Verification items for this drawing (mm, ordinates from the low corner). A direction names the side the tool comes from. Coordinates: 2 decimals unless noted, no trailing zeros. Loops run counter-clockwise (first coordinate to the right, second up) from the corner with the lowest first, then second, coordinate; pieces in that order, holes last. Notation, with made-up numbers: M 25,-33.75 L 43,-33.75 A16 ccw 43,-10.75 Z; hole C 66,-27 d6. An arc over 180 degrees is marked long. Return JSON: item names as keys, results as strings.
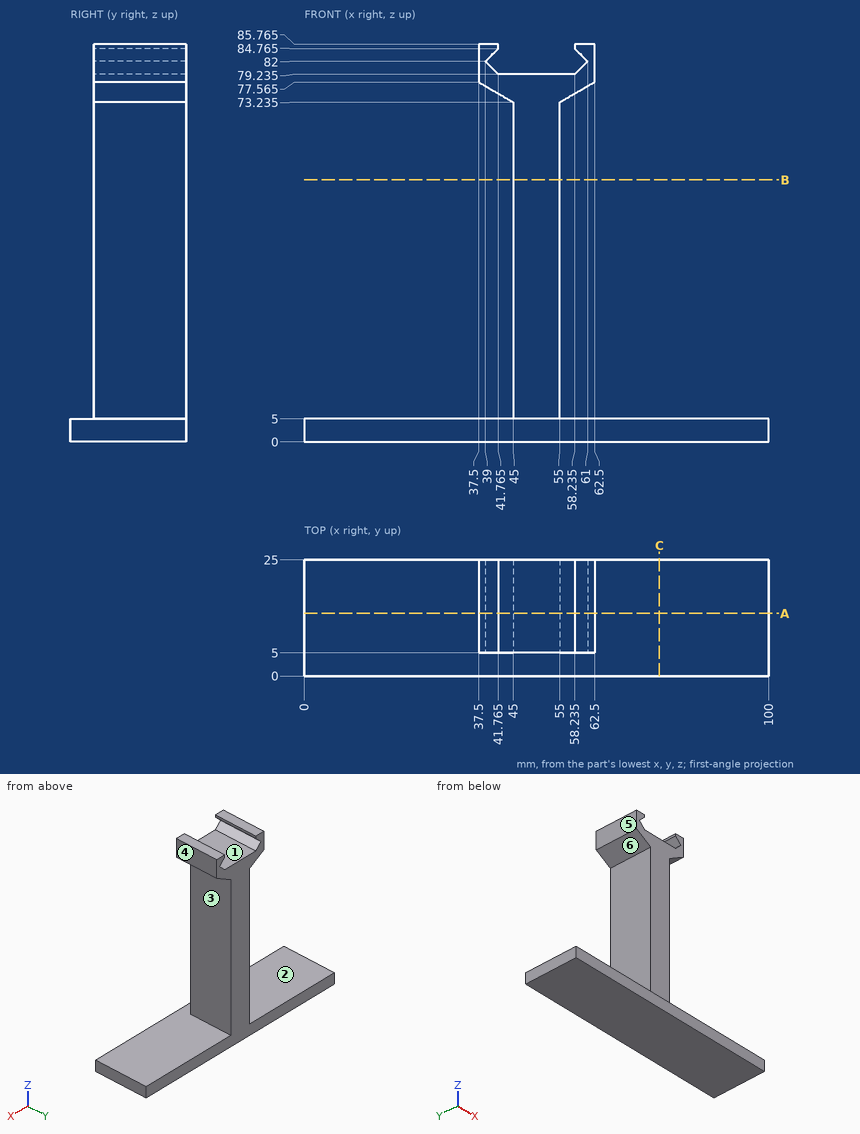
1) Section check A-A on y = 13.5. Record the cut outline in (x, z) (3 decimals).
Answers:
{"outline": "M 0,0 L 100,0 L 100,5 L 55,5 L 55,73.235 L 62.5,77.565 L 62.5,85.765 L 58.235,85.765 L 58.235,84.765 L 61,82 L 58.235,79.235 L 41.765,79.235 L 39,82 L 41.765,84.765 L 41.765,85.765 L 37.5,85.765 L 37.5,77.565 L 45,73.235 L 45,5 L 0,5 Z"}
2) Scan lines: line 1 along Y through (x, z) = (50, 62); line 2 along Z through (x, y) = (78, 22.25); line 3 along X through (y, z) = (9, 13.5). Record each from-to range of solid material in increasing order. Write a range as [from, to].
Answers:
{"line 1": "[5, 25]", "line 2": "[0, 5]", "line 3": "[45, 55]"}
3) Go/stop test with flat-tipped pins: pin 1 Ø6 at (y, z) = (21.5, 22.5) entering from +X; pin 2 Ø6 at (y, z) = (11, 76) entering from +X; pin 3 Ø0.5 at (y, z) = (11.5, 85.5) entering from -X. Record where each tip stops, or that it passes through.
Answers:
{"pin 1": "x = 55", "pin 2": "x = 62.5", "pin 3": "x = 37.5"}
4) Set-up check for the marked faces 4, 5 and 6: record each of +Z, -Z, +X, -X, +Y, -Y from which the full face is reachable in a straight line by a thin tool's end or side.
Answers:
{"face 4": "+Z, +X, +Y, -Y", "face 5": "+Z, -X, +Y, -Y", "face 6": "-X, +Y, -Y"}
5) Draft check along X on the marked faces 1, 2 and 3. Enter one of: +X half, -X half, draft (parallel to the pull), parting line (faces both ways), or undercut.
Answers:
{"face 1": "undercut", "face 2": "draft", "face 3": "+X half"}
6) Section check B-B on z = 56.5. Record the cut outline in (x, y), then the cut area to 3 significant figures.
Answers:
{"outline": "M 45,5 L 55,5 L 55,25 L 45,25 Z", "area": "200 mm²"}
7) Section check C-C on x = 76.5. Record the cut outline in (y, z).
Answers:
{"outline": "M 0,0 L 25,0 L 25,5 L 0,5 Z"}
